from build123d import *

# Parameters (mm, degrees)
F1_DEPTH      = 79
F3_DEPTH      = 14
F4_R          = 2.7
F5_DEPTH      = 79
F8_DEPTH      = 25
F8_DEPTH_BACK = 25


with BuildPart() as f1:
    # F0 (on Top) → F1 (new body)
    with BuildSketch(Plane.XY):
        Polygon((-9, 7), (-23, 7), (-23, -7), (-9, -7), (-9, -15), (9, -15), (9, -7), (23, -7), (23, 7), (9, 7), (9, 15), (-9, 15), align=None)
    extrude(amount=F1_DEPTH)

    # F2 (on face) → F3 (cut, through all)
    with BuildSketch(Plane.XZ.offset(7)):
        Polygon((-9, 39.5), (-23, 63), (-23, 16), align=None)
        Polygon((23, 63), (9, 39.5), (23, 16), align=None)
    extrude(amount=-F3_DEPTH, mode=Mode.SUBTRACT)

    # F4 (on face) → F5 (cut)
    with BuildSketch(Plane.XY.offset(79)):
        with Locations((-16, 0)):
            Circle(F4_R)
        with Locations((16, 0)):
            Circle(F4_R)
    extrude(amount=-F5_DEPTH, mode=Mode.SUBTRACT)

    # F7 (on offset) → F8 (cut, two sides)
    with BuildSketch(Plane.XY.offset(39.5)) as f8_sk:
        Polygon((-16, 4.9074772881), (-20.25, 2.4537386441), (-20.25, -2.4537386441), (-16, -4.9074772881), (-11.75, -2.4537386441), (-11.75, 2.4537386441), align=None)
        Polygon((20.25, -2.4537386441), (20.25, 2.4537386441), (16, 4.9074772881), (11.75, 2.4537386441), (11.75, -2.4537386441), (16, -4.9074772881), align=None)
    extrude(amount=-F8_DEPTH, mode=Mode.SUBTRACT)
    extrude(f8_sk.sketch, amount=F8_DEPTH_BACK, mode=Mode.SUBTRACT)


solid = f1.part
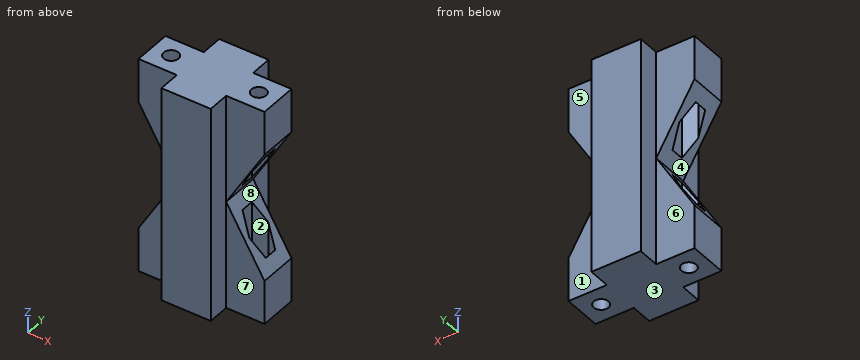
Check sheet for the modelled part. Datum: model origin and axes. Units: mm. Face numbers are marked on the shaded views. A direction names the side the tool comes from. Round coordinates to 2 decimals unless told otherwise and drop trailing zeros. Write each loop counter-clockwise with the first axis right and the second up, starting at its lowest first coordinate (ties: lowest second). Pieces come first, ordered by that corner, then holes. Notation, with made-up numbers: (68, -2.5) -> (84, -2.5) arc R29 ccw to (84, 25.5) -> close; hole circle Ø2 at (-30, 27). An arc over 180 degrees is marked (long way). Answer as CSV lines item,"result". Start each with the question number.
1) Material ranges on line 1 (Y direction, x = -16, z = 6); line 2 (Z direction, x = 20, y = 1.25); line 3 (X direction, y = 9.25, z = 26), recorded low to high. Write a range as from..to.
2) Section check D-D on y = 4. Enter the section's corners in (x, z).
3) Section check C-C on z = 52.5. Enter the section's corners in (x, y), and give its area (3 significant figures).
4) Section check A-A on z = 11. Enter the section's corners in (x, y), and give its area (3 significant figures).
5) Go/stop test with flat-tipped pins: P1, Ø5, axis at x = 18, z = 15.5, coming from the +Y side; P2, Ø1.5, axis at y = -1, z = 23, coming from the -X side; P3, Ø6.5, axis at y = 11, z = 24, coming from the -X side. Record where each tip stops, or that it passes through.
6) Section check B-B on x = -15. Enter the section's corners in (y, z).
7) Tool access check on the marked faces 4, 5, 6, 7 and 8. Record the directions out of +Z, -Z, +X, -X, +Y, -Y that give a thin tool (end or side, any length) a straight path to the whole face; none if there is none.
8) Release check for a two-part mould opening along Z. For the marked faces 1, 2 and 3 record: pulls with the +Z half, pulls with the -Z half, needs draft (parallel to the pull), parting line crosses it, or undercut.
Found:
1,line 1,"y = -7..-2.7, 2.7..7"
1,line 2,"z = 0..14.5, 64.5..79"
1,line 3,"x = -9..9"
2,outline,"(-23, 0) -> (23, 0) -> (23, 16) -> (17.57, 25.11) -> (17.57, 14.5) -> (14.43, 14.5) -> (14.43, 30.39) -> (9, 39.5) -> (14.43, 48.61) -> (14.43, 64.5) -> (17.57, 64.5) -> (17.57, 53.89) -> (23, 63) -> (23, 79) -> (-23, 79) -> (-23, 63) -> (-17.57, 53.89) -> (-17.57, 64.5) -> (-14.43, 64.5) -> (-14.43, 48.61) -> (-9, 39.5) -> (-14.43, 30.39) -> (-14.43, 14.5) -> (-17.57, 14.5) -> (-17.57, 25.11) -> (-23, 16) -> close"
3,outline,"(-16.74, -7) -> (-9, -7) -> (-9, -15) -> (9, -15) -> (9, -7) -> (16.74, -7) -> (16.74, -4.48) -> (16, -4.91) -> (11.75, -2.45) -> (11.75, 2.45) -> (16, 4.91) -> (16.74, 4.48) -> (16.74, 7) -> (9, 7) -> (9, 15) -> (-9, 15) -> (-9, 7) -> (-16.74, 7) -> (-16.74, 4.48) -> (-16, 4.91) -> (-11.75, 2.45) -> (-11.75, -2.45) -> (-16, -4.91) -> (-16.74, -4.48) -> close"
3,area,"680 mm^2"
4,outline,"(-23, -7) -> (-9, -7) -> (-9, -15) -> (9, -15) -> (9, -7) -> (23, -7) -> (23, 7) -> (9, 7) -> (9, 15) -> (-9, 15) -> (-9, 7) -> (-23, 7) -> close; hole circle Ø5.4 at (-16, 0); hole circle Ø5.4 at (16, 0)"
4,area,"886 mm^2"
5,P1,"stops at y = 7"
5,P2,"stops at x = -11.75"
5,P3,"stops at x = -9"
6,outline,"(-7, 0) -> (-2.51, 0) -> (-2.51, 14.5) -> (-4.33, 14.5) -> (-4.33, 29.43) -> (-7, 29.43) -> close; (-7, 49.57) -> (-4.33, 49.57) -> (-4.33, 64.5) -> (-2.51, 64.5) -> (-2.51, 79) -> (-7, 79) -> close; (2.51, 0) -> (7, 0) -> (7, 29.43) -> (4.33, 29.43) -> (4.33, 14.5) -> (2.51, 14.5) -> close; (2.51, 64.5) -> (4.33, 64.5) -> (4.33, 49.57) -> (7, 49.57) -> (7, 79) -> (2.51, 79) -> close"
7,face 4,"-X, +Y, -Y"
7,face 5,"+Z, -Z, +X, +Y"
7,face 6,"+Z, -Z, -X, +Y"
7,face 7,"+Z, -Z, +X, -Y"
7,face 8,"+X, +Y, -Y"
8,face 1,"needs draft"
8,face 2,"undercut"
8,face 3,"pulls with the -Z half"
